```python
from build123d import *

# Parameters (mm, degrees)
SCHIZZO1_W                   = 100
SCHIZZO1_H                   = 80
SCHIZZO1_R                   = 1.5
ESTRUSIONE_ESTRUSIONE1_DEPTH = 3
SCHIZZO2_W                   = 100
SCHIZZO2_H                   = 50
ESTRUSIONE_ESTRUSIONE2_DEPTH = 3
SCHIZZO3_W                   = 86
SCHIZZO3_H                   = 50
ESTRUSIONE_ESTRUSIONE3_DEPTH = 3


with BuildPart() as part:
    # Schizzo1 → Estrusione-Estrusione1 (new body)
    with BuildSketch(Plane(origin=(0, 0, 0), x_dir=(1, 0, 0), z_dir=(0, 1, 0))):
        with Locations((50, 40)):
            Rectangle(SCHIZZO1_W, SCHIZZO1_H)
        with Locations(Location((15, 67.4, 0), (0, 0, 270))):
            Circle(SCHIZZO1_R, mode=Mode.SUBTRACT)
        with Locations(Location((15, 12.6, 0), (0, 0, 90))):
            Circle(SCHIZZO1_R, mode=Mode.SUBTRACT)
        with Locations(Location((76.978953205, 59.25, 0), (0, 0, 270))):
            Circle(SCHIZZO1_R, mode=Mode.SUBTRACT)
        with Locations(Location((76.978953205, 20.75, 0), (0, 0, 90))):
            Circle(SCHIZZO1_R, mode=Mode.SUBTRACT)
    extrude(amount=ESTRUSIONE_ESTRUSIONE1_DEPTH)

    # Schizzo2 → Estrusione-Estrusione2 (add)
    with BuildSketch(Plane.XY):
        with Locations((50, 25)):
            Rectangle(SCHIZZO2_W, SCHIZZO2_H)
    estrusione_estrusione2 = extrude(amount=ESTRUSIONE_ESTRUSIONE2_DEPTH)

    # Specchia1: Estrusione-Estrusione2 across plane
    add(estrusione_estrusione2.mirror(Plane.XY.offset(-40)))

    # Schizzo3 → Estrusione-Estrusione3 (add)
    with BuildSketch(Plane.ZY):
        with Locations((-40, 25)):
            Rectangle(SCHIZZO3_W, SCHIZZO3_H)
    extrude(amount=ESTRUSIONE_ESTRUSIONE3_DEPTH)


solid = part.part
```
Can you work these out from the model? Positions are in its coordinate system, mm. A direction names the side the tool comes from. Coordinates: 2 decimals unless noted, no trailing zeros. Order: outer loops, then holes, each group sorted by start corner. A loop starts at its lowest first (then second) coordinate and runs counter-clockwise, first axis right, second up. Notation, with made-up numbers: (87, 8.5) - (95, 8.5) arc R20 ccw to (95, 32.5) - close; hole circle Ø7 at (30.5, 3). An arc over 180 degrees is marked (long way). Answer in a Markdown table with one row per item.
1. If I drill on line 1 along Z through (x, y) = (63.5, 43.5); line 2 along X through (y, z) = (1, -59); line 3 along X through (y, z) = (0.85, -12.6), over which ranges is the centre line in solid material (lowest first)?
Reply:
| item | result |
|---|---|
| line 1 | z = -83 to -80, 0 to 3 |
| line 2 | x = -3 to 75.5, 78.46 to 100 |
| line 3 | x = -3 to 13.5, 16.5 to 100 |
2. Suppose I cut it at B-B (x = 15). Please give me the cut outline in (y, z), and give its area (3 significant figures).
Reply:
| item | result |
|---|---|
| outline | (0, -83) - (50, -83) - (50, -80) - (3, -80) - (3, -68.9) - (0, -68.9) - close; (0, -65.9) - (3, -65.9) - (3, -14.1) - (0, -14.1) - close; (0, -11.1) - (3, -11.1) - (3, 0) - (50, 0) - (50, 3) - (0, 3) - close |
| area | 522 mm^2 |
3. Suppose I cut it at C-C (y = 6). Please give me the cut outline in (x, z).
Reply:
| item | result |
|---|---|
| outline | (-3, -83) - (100, -83) - (100, -80) - (0, -80) - (0, 0) - (100, 0) - (100, 3) - (-3, 3) - close |
4. Suppose I cut it at D-D (z = -34.5). Please give me the cut outline in (x, y), and give its area (3 significant figures).
Reply:
| item | result |
|---|---|
| outline | (-3, 0) - (100, 0) - (100, 3) - (0, 3) - (0, 50) - (-3, 50) - close |
| area | 450 mm^2 |
5. For faces 4 (the cylindrical face through (15.45, 1.48, -65.97)), 5 (the flat face through (0, 27, -41)), which set-ups out of +Z, -Z, +X, -X, +Y, -Y let a thin tool reach every point of the face, with its end or its side?
Reply:
| item | result |
|---|---|
| face 4 | +Y, -Y |
| face 5 | +X, +Y |
6. If we mould it in two halves opening along X, with no side actions, what happens to faces 1 (the cylindrical face through (77.43, 1.48, -57.82)), 2 (the flat face through (49, 25, -83)), 3 (the flat face through (-3, 25, -41))? For each: pulls with the +X half, pulls with the -X half, needs draft (parallel to the pull), parting line crosses it, or undercut.
Reply:
| item | result |
|---|---|
| face 1 | undercut |
| face 2 | needs draft |
| face 3 | pulls with the -X half |
7. Suppose I cut it at A-A (z = -59.25). Please give me the cut outline in (x, y), and give its area (3 significant figures).
Reply:
| item | result |
|---|---|
| outline | (-3, 0) - (75.48, 0) - (75.48, 3) - (0, 3) - (0, 50) - (-3, 50) - close; (78.48, 0) - (100, 0) - (100, 3) - (78.48, 3) - close |
| area | 441 mm^2 |
8. For pin 1 (1.8 mm diameter, centred on x = 76.98, z = -20.75, fed in from -Y); pin 2 (3.5 mm diameter, centred on x = 76.98, z = -59.25, fed in from +Y); pin 3 (23.5 mm diameter, centred on y = 16, z = -48, fed in from +X), each with a flat end and sliding along its axis, tell me the tip position at first contact or that it passes through.
Reply:
| item | result |
|---|---|
| pin 1 | passes through |
| pin 2 | stops at y = 3 |
| pin 3 | stops at x = 0 |
